Can you work these out from the model? Positions are in its coordinate system, mm. A direction names the side the tool comes from. Round coordinates to 2 decimals unless told otherwise and drop trailing zeros. Write each loop counter-clockwise with the first axis right and the second up, starting at its lowest first coordinate (ties: lowest second). Pieces come first, ordered by that corner, then holes. Notation, with made-up numbers: M 61.5,11.5 L 116.5,11.5 A25 ccw 116.5,37.5 Z; hole C 17,6 d11. An arc over 180 degrees is marked long. Answer in a Markdown table with one row per item. Add a question column.
(1) Suppose I cut it at D-D, the plane z = -31.5. Write out the boundary of the cut face in (x, y), then the cut area to 3 significant figures.
(2) I'm going to push flat-ended pins straight in: pin 1 (8 mm diameter, centred on x = -36, y = 143.5, fed in from +Z); pin 2 (5 mm diameter, centred on x = -15, y = 32.5, fed in from +Z); pin 3 (3.5 mm diameter, centred on x = -16, y = 146.5, fed in from -Z). Where does each tip first touch, or does it pass through?
(3) Suppose I cut it at B-B, the plane y = 41.5. Write out the boundary of the cut face in (x, z).
(4) For faces 5 (the face through (-29.278, 145.07, 7.986)), 6 (the face through (1, 150, 1)), which set-ups out of +Z, -Z, +X, -X, +Y, -Y let a thin tool reach every point of the face, with its end or its side?
(5) Suppose I cut it at A-A, the plane x = -9.5. Write out the boundary of the cut face in (y, z), then the cut area to 3 significant figures.
(6) Suppose I cut it at C-C, the plane z = 40. Write out the boundary of the cut face in (x, y).
(7) If we mould it in two halves opening along Z, with no side actions, what happens to faces 1 (the face through (1, 0, 1)), 2 (the face through (-34, 145, -17.364)), 3 (the face through (-23.5, 140, 5.7)), 4 (the face through (-62, 73.95, -19.52))? For each: released by +Z, released by -Z, zero draft, split by the parting line, or undercut.
(8) If I drill on probe 1 along Y at (x, z) = (-13, 16.5); probe 2 along X at (y, z) = (58, -11.5); probe 3 along X at (y, z) = (69.5, -48), over which ranges is the centre line in solid material (lowest first)?
Autodesk Inventor part; units mm, degrees
ref_plane "YZ Plane" through (0, 0, 0) normal (1, 0, 0) x (0, 1, 0)
ref_plane "XZ Plane" through (0, 0, 0) normal (0, 1, 0) x (-1, 0, 0)
ref_plane "XY Plane" through (0, 0, 0) normal (0, 0, 1) x (1, 0, 0)
sketch "Sketch1" plane through (0, 0, 0) normal (0, 1, 0) x (-1, 0, 0)
  circle A0 centre (0, 0) radius 65
  line L0 (0, 0) -> (0, -25) construction
  circle A1 centre (0, -25) radius 11.5 construction
  circle A2 centre (21.6506, -12.5) radius 11.5 construction
  circle A3 centre (21.6506, 12.5) radius 11.5 construction
  circle A4 centre (0, 25) radius 11.5 construction
  circle A5 centre (-21.6506, 12.5) radius 11.5 construction
  circle A6 centre (-21.6506, -12.5) radius 11.5 construction
  line L1 (0, 0) -> (-21.6506, 37.5) construction
  circle A7 centre (-21.6506, 37.5) radius 11.5 construction
  circle A8 centre (-43.3013, 0) radius 11.5 construction
  circle A9 centre (-21.6506, -37.5) radius 11.5 construction
  circle A10 centre (21.6506, -37.5) radius 11.5 construction
  circle A11 centre (43.3013, 0) radius 11.5 construction
  circle A12 centre (21.6506, 37.5) radius 11.5 construction
  circle A13 centre (0, 50) radius 11.5 construction
  circle A14 centre (-43.3013, 25) radius 11.5 construction
  circle A15 centre (-43.3013, -25) radius 11.5 construction
  circle A16 centre (0, -50) radius 11.5 construction
  circle A17 centre (43.3013, -25) radius 11.5 construction
  circle A18 centre (43.3013, 25) radius 11.5 construction
  dimension "d0" = 130
  dimension "d5" = 25
  dimension "d6" = 23
  dimension "d9" = 360
  dimension "d11" = 23
  dimension "d13" = 150
  dimension "d16" = 360
  dimension "d18" = 25
  dimension "d19" = 25
  dimension "d20" = 25
  dimension "d21" = 25
  dimension "d22" = 23
  dimension "d25" = 360
extrude "Extrusion1" add sketch "Sketch1" along normal blind 150
sketch "Sketch2" plane through (0, 150, 0) normal (0, 1, 0) x (1, 0, 0)
  line L0 (-37.7255, 18.2555) -> (-21.2587, 18.2555) construction
  line L1 (-21.2587, 18.2555) -> (-21.2587, 7.8989) construction
  line L2 (-21.2587, 7.8989) -> (-37.7255, 7.8989) construction
  line L3 (-37.7255, 7.8989) -> (-37.7255, 18.2555) construction
  line L4 (3.6035, 17.3641) -> (-13.6169, -32.6359)
  line L5 (-13.6169, -32.6359) -> (-20.7887, -32.6359)
  line L6 (-20.7887, -32.6359) -> (-38.0091, 17.3641)
  line L7 (-38.0091, 17.3641) -> (-30.8779, 17.3641)
  line L8 (-30.8779, 17.3641) -> (-17.0205, -24.1675)
  line L9 (-17.0205, -24.1675) -> (-3.1631, 17.3641)
  line L10 (-3.1631, 17.3641) -> (3.6035, 17.3641)
  spline S0 degree 2 poles (27.9147, -33.5273) (23.0524, -33.5273) (14.8272, -30.2453) (11.8288, -26.9633) knots 0 0 0 1 2 2 2
  spline S1 degree 2 poles (11.8288, -26.9633) (8.8304, -23.7218) (5.5484, -13.9973) (5.5484, -7.6764) knots 0 0 0 1 2 2 2
  spline S2 degree 2 poles (5.5484, -7.6764) (5.5484, -1.396) (8.7494, 7.9232) (11.7883, 11.3673) knots 0 0 0 1 2 2 2
  spline S3 degree 2 poles (11.7883, 11.3673) (14.7866, 14.7304) (22.9714, 18.2555) (28.0362, 18.2555) knots 0 0 0 1 2 2 2
  spline S4 degree 2 poles (28.0362, 18.2555) (30.5484, 18.2555) (34.9649, 17.5262) (36.8288, 16.9589) knots 0 0 0 1 2 2 2
  spline S5 degree 2 poles (36.8288, 16.9589) (38.4495, 16.4322) (41.8126, 14.933) (43.4738, 14.0416) knots 0 0 0 1 2 2 2
  line L11 (43.4738, 14.0416) -> (43.4738, 6.0189)
  line L12 (43.4738, 6.0189) -> (42.9471, 6.0189)
  spline S6 degree 2 poles (42.9471, 6.0189) (42.0557, 6.8292) (39.3004, 9.0983) (37.315, 10.1923) knots 0 0 0 1 2 2 2
  spline S7 degree 2 poles (37.315, 10.1923) (35.4106, 11.2458) (30.9131, 12.5829) (27.9957, 12.5829) knots 0 0 0 1 2 2 2
  spline S8 degree 2 poles (27.9957, 12.5829) (24.7947, 12.5829) (19.0816, 9.9492) (16.9341, 7.437) knots 0 0 0 1 2 2 2
  spline S9 degree 2 poles (16.9341, 7.437) (14.8272, 4.8843) (12.4771, -2.8547) (12.4771, -7.6764) knots 0 0 0 1 2 2 2
  spline S10 degree 2 poles (12.4771, -7.6764) (12.4771, -12.8223) (14.9487, -20.2372) (17.0962, -22.7899) knots 0 0 0 1 2 2 2
  spline S11 degree 2 poles (17.0962, -22.7899) (19.2032, -25.2615) (24.8353, -27.7737) (27.9957, -27.7737) knots 0 0 0 1 2 2 2
  spline S12 degree 2 poles (27.9957, -27.7737) (30.8725, -27.7737) (35.7753, -26.3555) (37.6797, -25.302) knots 0 0 0 1 2 2 2
  spline S13 degree 2 poles (37.6797, -25.302) (39.503, -24.2486) (42.2178, -22.0606) (42.9876, -21.2907) knots 0 0 0 1 2 2 2
  line L13 (42.9876, -21.2907) -> (43.4738, -21.2907)
  line L14 (43.4738, -21.2907) -> (43.4738, -29.2324)
  spline S14 degree 2 poles (43.4738, -29.2324) (41.8126, -30.0022) (38.8952, -31.4204) (36.8288, -32.0687) knots 0 0 0 1 2 2 2
  spline S15 degree 2 poles (36.8288, -32.0687) (34.6408, -32.798) (30.9131, -33.5273) (27.9147, -33.5273) knots 0 0 0 1 2 2 2
  point P0 (0, 0)
extrude "Extrusion2" cut sketch "Sketch2" against normal blind 10
equation "\"d11\" = d6"
equation "\"d21\" = d19"
equation "\"d22\" = d6"
properties part number "VialCarousel"
Calculated:
| question | item | result |
|---|---|---|
| 1 | outline | M -56.86,0 L 56.86,0 L 56.86,150 L -56.86,150 Z |
| 1 | area | 17,100 mm² |
| 2 | pin 1 | z = 56.58 |
| 2 | pin 2 | z = 63.79 |
| 2 | pin 3 | z = -63.42 |
| 3 | outline | C 0,0 d130 |
| 4 | face 5 | +Y |
| 4 | face 6 | +Z, -Z, +X, -X, +Y |
| 5 | outline | M 0,-64.3 L 150,-64.3 L 150,1.63 L 140,1.63 L 140,20.68 L 150,20.68 L 150,64.3 L 0,64.3 Z |
| 5 | area | 19,100 mm² |
| 6 | outline | M -51.23,0 L 51.23,0 L 51.23,150 L -51.23,150 Z |
| 7 | face 1 | zero draft |
| 7 | face 2 | undercut |
| 7 | face 3 | undercut |
| 7 | face 4 | split by the parting line |
| 8 | probe 1 | 0 to 140 |
| 8 | probe 2 | -63.97 to 63.97 |
| 8 | probe 3 | -43.83 to 43.83 |
